from build123d import *

# Parameters (mm, degrees)
SKETCH1_W           = 13
SKETCH1_H           = 20
BOSS_EXTRUDE1_DEPTH = 3
SKETCH2_W           = 3
SKETCH2_H           = 2
SKETCH2_H_2         = 3
CUT_EXTRUDE1_DEPTH  = 3
SKETCH3_W           = 3
SKETCH3_H           = 2
SKETCH3_H_2         = 3
CUT_EXTRUDE2_DEPTH  = 3


with BuildPart() as part:
    # Sketch1 → Boss-Extrude1 (new body)
    with BuildSketch(Plane.XY):
        Rectangle(SKETCH1_W, SKETCH1_H)
    extrude(amount=BOSS_EXTRUDE1_DEPTH)

    # Sketch2 → Cut-Extrude1 (cut)
    with BuildSketch(Plane.XY.offset(3)):
        with Locations((-5, 9)):
            Rectangle(SKETCH2_W, SKETCH2_H)
        with Locations((-5, 5)):
            Rectangle(SKETCH2_W, SKETCH2_H_2)
        with Locations((-5, 0.5)):
            Rectangle(SKETCH2_W, SKETCH2_H_2)
        with Locations((-5, -4)):
            Rectangle(SKETCH2_W, SKETCH2_H_2)
        with Locations((-5, -8.5)):
            Rectangle(SKETCH2_W, SKETCH2_H_2)
    extrude(amount=-CUT_EXTRUDE1_DEPTH, mode=Mode.SUBTRACT)

    # Sketch3 → Cut-Extrude2 (cut)
    with BuildSketch(Plane.XY.offset(3)):
        with Locations((5, 9)):
            Rectangle(SKETCH3_W, SKETCH3_H)
        with Locations((5, 5)):
            Rectangle(SKETCH3_W, SKETCH3_H_2)
        with Locations((5, 0.5)):
            Rectangle(SKETCH3_W, SKETCH3_H_2)
        with Locations((5, -4)):
            Rectangle(SKETCH3_W, SKETCH3_H_2)
        with Locations((5, -8.5)):
            Rectangle(SKETCH3_W, SKETCH3_H_2)
    extrude(amount=-CUT_EXTRUDE2_DEPTH, mode=Mode.SUBTRACT)


solid = part.part
Design review of the part built by this model. Coordinates are the model's own, in mm. A direction names the side the tool comes from. Coordinates: 2 decimals unless noted, no trailing zeros. Order: outer loops, then holes, each group sorted by start corner. A loop starts at its lowest first (then second) coordinate and runs counter-clockwise, first axis right, second up. Notation, with made-up numbers: (16.5, 85) -> (55.5, 85) arc R28 cw to (55.5, 115) -> close; hole circle Ø8 at (-29.5, 72). An arc over 180 degrees is marked (long way). Use one line per item in the form item = value. Start each with the question number.
(1) Insertion check: pin 1 (0.9 mm diameter, centred on x = -5, z = 2, fed in from +Y); pin 2 (1.5 mm diameter, centred on x = -5, z = 2, fed in from -Y). Each pin has a flat end and moves straight along its axis. Give the tip position at first contact, or say it passes through.
(2) The part is to be moulded in two halves that separate along Y. For faces 1 (the flat face through (-5, 8, 2)), 2 (the flat face through (-5, -2.5, 2)), 3 (the flat face through (-5, -7, 2)), say which applies: +Y half, -Y half, draft (parallel to the pull), parting line (faces both ways), or undercut.
(3) For faces 4 (the flat face through (5, 8, 2)), 5 (the flat face through (5, -2.5, 2)), 6 (the flat face through (-3.5, 5, 2)), list the 3-axis set-ups (+Z, -Z, +X, -X, +Y, -Y) from which the entire face can be reached by the end or side of a thin tool; tool diameter is ignored.
(4) For probe 1 along Y at (x, z) = (-5.5, 0.5); probe 2 along X at (y, z) = (-4.25, 2.45), list the stretches that pass through material, from the lowest coordinate up.
(5) Add section B-B on y = 6. State the section outline as (x, z) points, plus the area to 3 significant figures.
(6) Add section A-A on x = 4.5. State the section outline as (y, z) points, plus the area to 3 significant figures.
Answer block:
q1.pin_1 = 8
q1.pin_2 = -7
q2.face_1 = +Y half
q2.face_2 = undercut
q2.face_3 = -Y half
q3.face_4 = +Z, -Z, +X, +Y
q3.face_5 = +Z, -Z, +X
q3.face_6 = +Z, -Z, -X
q4.probe_1 = -7 to -5.5, -2.5 to -1, 2 to 3.5, 6.5 to 8
q4.probe_2 = -3.5 to 3.5
q5.outline = (-3.5, 0) -> (3.5, 0) -> (3.5, 3) -> (-3.5, 3) -> close
q5.area = 21.0 mm²
q6.outline = (-7, 0) -> (-5.5, 0) -> (-5.5, 3) -> (-7, 3) -> close; (-2.5, 0) -> (-1, 0) -> (-1, 3) -> (-2.5, 3) -> close; (2, 0) -> (3.5, 0) -> (3.5, 3) -> (2, 3) -> close; (6.5, 0) -> (8, 0) -> (8, 3) -> (6.5, 3) -> close
q6.area = 18.0 mm²
